Answer from the drawing. Dimensions are ordinates in mm from the lowest x, y and z of the part. Coordinates: 2 decimals unless noted, no trailing zeros. Loops run counter-clockwise (first coordinate to the right, second up) from the corner with the lowest first, then second, coordinate; pieces in that order, holes last. Notation, with made-up numbers: (-36.75, 0.25) - (-13.75, 0.25) arc R9 ccw to (-13.75, 10.25) - close; hole circle Ø3 at (-9, 82.5). An arc over 180 degrees is marked (long way). Use one line per item in the form item = value. Start each with the question number.
1) Each of these flat-tipped pins is pushed along its axis until it touches: P1, Ø2, axis at y = 2, z = 26.5, coming from the -X side; P2, Ø1.5, axis at x = 36.5, y = 4.5, coming from the +Z side; P3, Ø1, axis at x = 110.5, y = 3.5, coming from the -Z side (1 decimal); P4, Ø3.5, axis at x = 63.5, z = 63.5, coming from the -Y side. Where does it stop, or does it pass through?
2) A cutting plane is placed at A-A (y = 5). Give the vertices of the cut face in (x, z) (1 decimal), and give its area (3 significant figures).
3) A cutting plane is placed at B-B (x = 57). Give the vertices of the cut face in (y, z).
4) A cutting plane is placed at C-C (z = 22). Give the vertices of the cut face in (x, y).
5) A cutting plane is placed at D-D (x = 113.5). Give the vertices of the cut face in (y, z).
6) Consider line 1 (X direction, y = 3, z = 63.5); line 2 (X direction, y = 5.25, z = 72.5) (1 decimal); line 3 (Z direction, x = 86, y = 1.5) (1 decimal). Determine where each line is inside the solid, lowest interval first.
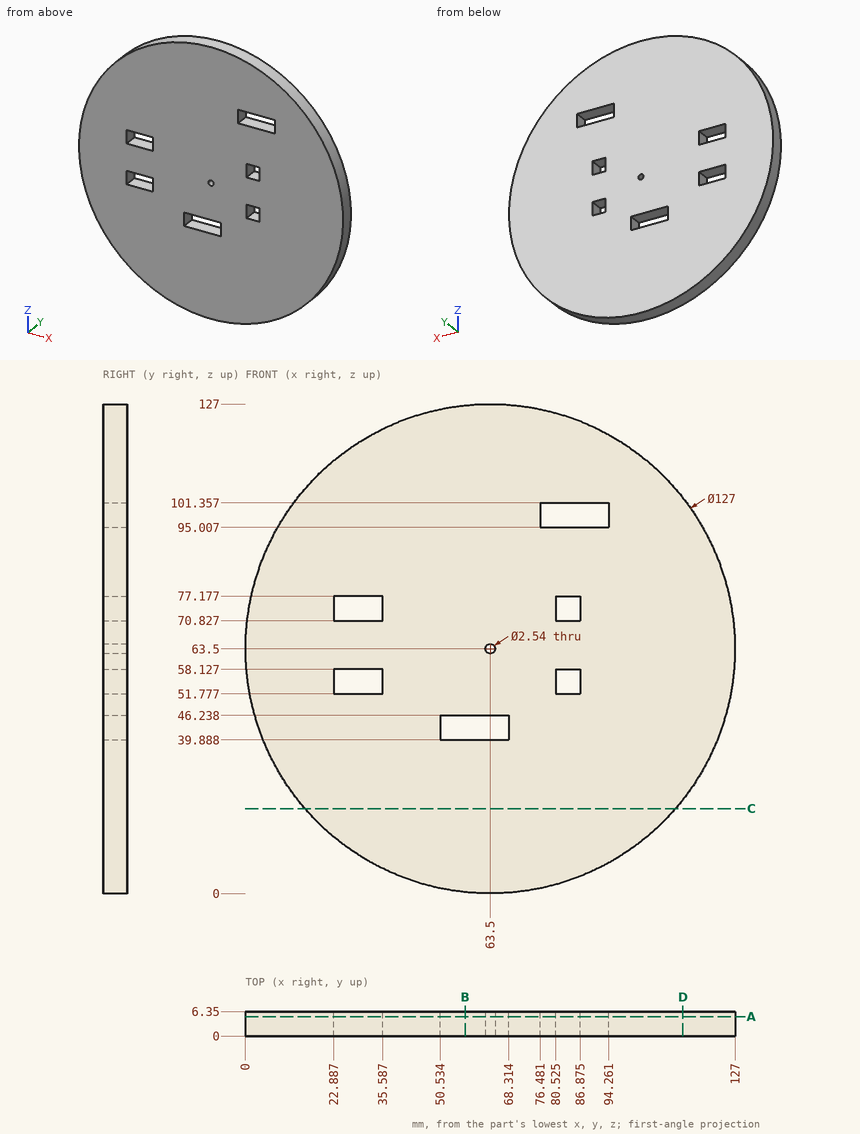
Found:
q1.P1 = 11.19
q1.P2 = 121.32
q1.P3 = 20.3
q1.P4 = 0
q2.outline = circle Ø127 at (63.5, 63.5); hole (22.9, 51.8) - (35.6, 51.8) - (35.6, 58.1) - (22.9, 58.1) - close; hole (22.9, 70.8) - (35.6, 70.8) - (35.6, 77.2) - (22.9, 77.2) - close; hole (50.5, 39.9) - (68.3, 39.9) - (68.3, 46.2) - (50.5, 46.2) - close; hole circle Ø2.5 at (63.5, 63.5); hole (76.5, 95) - (94.3, 95) - (94.3, 101.4) - (76.5, 101.4) - close; hole (80.5, 51.8) - (86.9, 51.8) - (86.9, 58.1) - (80.5, 58.1) - close; hole (80.5, 70.8) - (86.9, 70.8) - (86.9, 77.2) - (80.5, 77.2) - close
q2.area = 12,200 mm^2
q3.outline = (0, 0.33) - (6.35, 0.33) - (6.35, 39.89) - (0, 39.89) - close; (0, 46.24) - (6.35, 46.24) - (6.35, 126.67) - (0, 126.67) - close
q4.outline = (15.44, 0) - (111.56, 0) - (111.56, 6.35) - (15.44, 6.35) - close
q5.outline = (0, 24.36) - (6.35, 24.36) - (6.35, 102.64) - (0, 102.64) - close
q6.line_1 = 0 to 62.23, 64.77 to 127
q6.line_2 = 0.6 to 22.9, 35.6 to 80.5, 86.9 to 126.4
q6.line_3 = 4.1 to 51.8, 58.1 to 70.8, 77.2 to 95, 101.4 to 122.9
